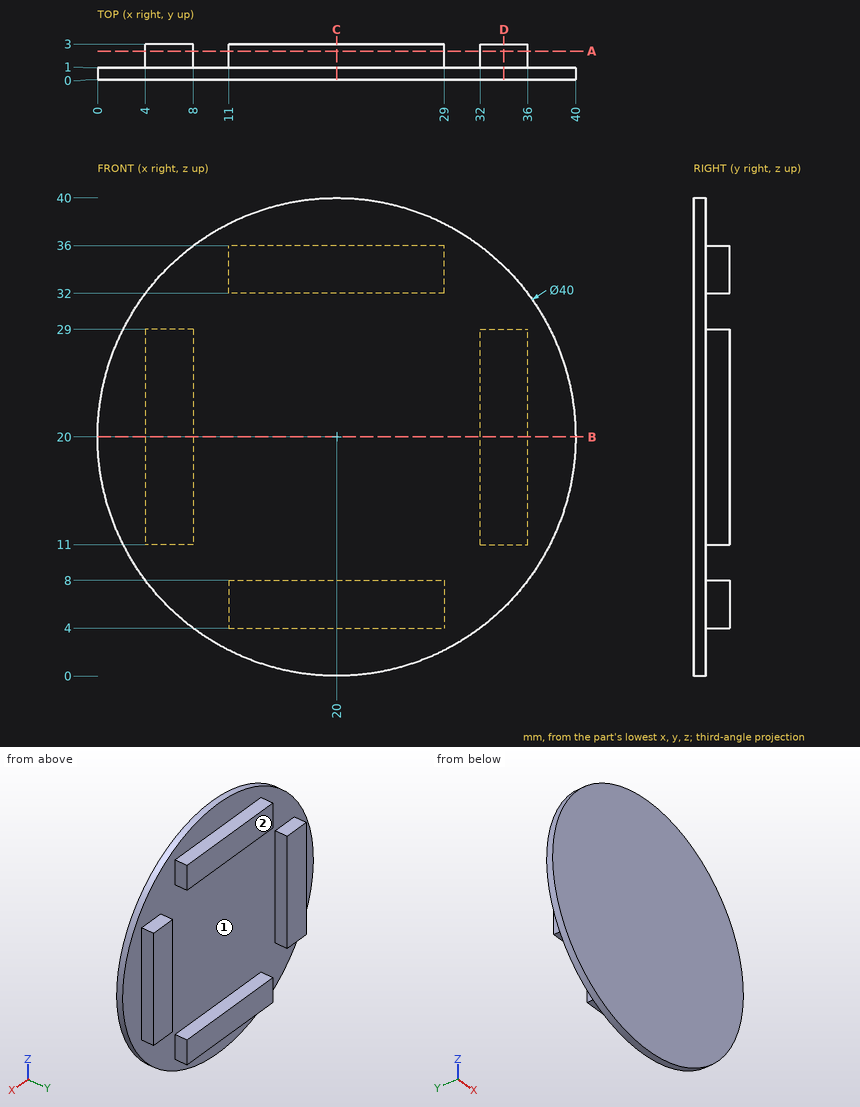
Could you check a few things on this drawing? It's one solid part, dimensions in mm from its lowest x, y, z. Round coordinates to 2 decimals unless told otherwise and drop trailing zeros. Write each loop counter-clockwise with the first axis right and the second up, starting at its lowest first coordinate (ties: lowest second). Pieces come first, ordered by that corner, then holes.
Q1. Please list where these lines run through material, in increasing order: probe 1 along Z at (x, y) = (24, 2.2); probe 2 along X at (y, z) = (1.65, 7.5).
Q2. If we section it at C-C on x = 20: Write out the boundary of the cut face in (y, z), plus the area to 3 significant figures.
Q3. If we section it at D-D on x = 34: Write out the boundary of the cut face in (y, z), plus the area to 3 significant figures.
Q4. If we mould it in two halves opening along Z, with no side actions, what happens to the marked faces 1 and 2? For each: +Z half, -Z half, draft (parallel to the pull), parting line (faces both ways), or undercut.
Q5. Will these pins go through, and if not, where does the flat tip stop? P1, Ø0.6, axis at y = 2, z = 17.5, coming from the -X side; P2, Ø1.6, axis at y = 2, z = 6, coming from the +X side; P3, Ø1.6, axis at y = 2, z = 20.5, coming from the +X side; P4, Ø5, axis at x = 20.5, z = 21.5, coming from the -Y side.
Q6. If we section it at B-B on z = 20: Write out the boundary of the cut face in (x, y).
Q7. If we section it at A-A on y = 2.4: Write out the boundary of the cut face in (x, z).
Answer below:
1. probe 1: z = 4 to 8, 32 to 36
1. probe 2: x = 11 to 29
2. outline: (0, 0) - (1, 0) - (1, 4) - (3, 4) - (3, 8) - (1, 8) - (1, 32) - (3, 32) - (3, 36) - (1, 36) - (1, 40) - (0, 40) - close
2. area: 56.0 mm2
3. outline: (0, 5.72) - (1, 5.72) - (1, 11) - (3, 11) - (3, 29) - (1, 29) - (1, 34.28) - (0, 34.28) - close
3. area: 64.6 mm2
4. face 1: undercut
4. face 2: draft
5. P1: stops at x = 4
5. P2: stops at x = 29
5. P3: stops at x = 36
5. P4: stops at y = 0
6. outline: (0, 0) - (40, 0) - (40, 1) - (36, 1) - (36, 3) - (32, 3) - (32, 1) - (8, 1) - (8, 3) - (4, 3) - (4, 1) - (0, 1) - close
7. outline: (4, 11) - (8, 11) - (8, 29) - (4, 29) - close; (11, 4) - (29, 4) - (29, 8) - (11, 8) - close; (11, 32) - (29, 32) - (29, 36) - (11, 36) - close; (32, 11) - (36, 11) - (36, 29) - (32, 29) - close
